Source: CAD feature listing. Evaluate the final solid. Frame: model axes, mm. A direction names the side the tool comes from. Coordinates: 2 decimals unless noted, no trailing zeros. Loops run counter-clockwise (first coordinate to the right, second up) from the corner with the lowest first, then second, coordinate; pieces in that order, holes last. Notation, with made-up numbers: M 24.25,-7.5 L 67.25,-7.5 A20 cw 67.25,8.5 Z; hole C 84.5,-22 d9. An arc over 180 degrees is marked long. One line per question, with ' | ' between items. Start each with the question number.
1. Section query B-B, the plane y = 13.15. Output: boundary loops of the cut face in (x, z) (3 decimals), and give its area (3 significant figures).
2. Pin query (flat end, axial travel): P1, Ø1.5, axis at x = -18, z = 18.5, coming from the +Y side; P2, Ø22.5, axis at x = 8.5, z = 4.5, coming from the +Y side; P3, Ø12, axis at x = -4.5, y = 71, coming from the +Z side. Return the tip coordinate at first contact, or that it passes through.
3. Section query C-C, the plane x = 25. Output: boundary loops of the cut face in (y, z) (3 decimals), and give its area (3 significant figures).
4. Section query A-A, the plane z = 7.5. Output: boundary loops of the cut face in (x, y).
5. Ray query, probe 1 along Z at (x, y) = (24.5, 22.4) (3 decimals); probe 2 along Y at (x, z) = (24.5, 0); probe 3 along Z at (x, y) = (33, 13). Return the intervals inside material, ascending.
6. Access query for faces 4 (the flat face through (20.3, 17, 10)), 5 (the flat face through (33, 25.4, 12)), 6 (the flat face through (15, 15, 10)), 7 (the flat face through (10, 127.3, 60)), 8 (the flat face through (-14, 16, 18)). Directions: +Z, -Z, +X, -X, +Y, -Y. A direction counts if a zero-diameter tool reaches every point of the face in a straight line with its end or side. Return the directions, or none.
7. Mould query, pull axis Z, two halves, no side actions, for faces 1 (the flat face through (10.3, 17, 10)), 2 (the flat face through (10, 65, 45)), 3 (the flat face through (-28, 8, 2)). Classes: pulls with the +Z half, pulls with the -Z half, needs draft (parallel to the pull), parting line crosses it, or undercut.
8. Section query D-D, the plane z = 25.5. Output: boundary loops of the cut face in (x, y), and give its area (3 significant figures).
```python
from build123d import *

# Parameters (mm, degrees)
SKETCH1_R           = 1.5
BOSS_EXTRUDE1_DEPTH = 5
BOSS_EXTRUDE2_START = 5
SKETCH1_4_R         = 1.5
BOSS_EXTRUDE2_DEPTH = 10.3
BOSS_EXTRUDE3_START = 15.3
SKETCH1_5_W         = 10.3
SKETCH1_5_H         = 5
SKETCH1_5_R         = 1.5
BOSS_EXTRUDE3_DEPTH = 5
SKETCH2_W           = 28
SKETCH2_H           = 16
SKETCH2_R           = 1.625
BOSS_EXTRUDE4_DEPTH = 5
BOSS_EXTRUDE5_START = 15.35
SKETCH2_2_W         = 28
SKETCH2_2_H         = 16
SKETCH2_2_R         = 1.625
BOSS_EXTRUDE5_DEPTH = 5
CUT_EXTRUDE1_START  = 127.3
SKETCH3_R           = 3.81
CUT_EXTRUDE1_DEPTH  = 12.7
BOSS_EXTRUDE6_START = 20.3
SKETCH1_6_R         = 1.5
BOSS_EXTRUDE6_DEPTH = 25
BOSS_EXTRUDE7_START = 10.3
SKETCH1_7_W         = 10.3
SKETCH1_7_H         = 3.4
BOSS_EXTRUDE7_DEPTH = 5
BOSS_EXTRUDE8_DEPTH = 20


with BuildPart() as part:
    # Sketch1 → Boss-Extrude1 (new body)
    with BuildSketch(Plane(origin=(0, 0, 0), x_dir=(0, 0, -1), z_dir=(1, 0, 0))):
        Polygon((-15.35, 0), (-15.35, 23.4), (-5.05, 23.4), (-5.05, 0), (5, 0), (5, 35.4), (-30, 35.4), (-30, 140), (-75, 140), (-75, 127.3), (-45, 127.3), (-45, 0), align=None)
        with Locations((-0.195, 2.4)):
            Circle(SKETCH1_R, mode=Mode.SUBTRACT)
        with Locations((-0.195, 22.4)):
            Circle(SKETCH1_R, mode=Mode.SUBTRACT)
        with Locations((-20.195, 22.4)):
            Circle(SKETCH1_R, mode=Mode.SUBTRACT)
        with Locations((-20.195, 2.4)):
            Circle(SKETCH1_R, mode=Mode.SUBTRACT)
    extrude(amount=BOSS_EXTRUDE1_DEPTH)

    # Sketch1<4> → Boss-Extrude2 (add)
    with BuildSketch(Plane(origin=(0, 0, 0), x_dir=(0, 0, -1), z_dir=(1, 0, 0)).offset(BOSS_EXTRUDE2_START)):
        Polygon((-5.05, 0), (5, 0), (5, 25.4), (-30, 25.4), (-30, 140), (-75, 140), (-75, 127.3), (-45, 127.3), (-45, 0), (-15.35, 0), (-15.35, 23.4), (-5.05, 23.4), align=None)
        with Locations((-0.195, 22.4)):
            Circle(SKETCH1_4_R, mode=Mode.SUBTRACT)
        with Locations((-0.195, 2.4)):
            Circle(SKETCH1_4_R, mode=Mode.SUBTRACT)
        with Locations((-20.195, 2.4)):
            Circle(SKETCH1_4_R, mode=Mode.SUBTRACT)
        with Locations((-20.195, 22.4)):
            Circle(SKETCH1_4_R, mode=Mode.SUBTRACT)
    extrude(amount=BOSS_EXTRUDE2_DEPTH)

    # Sketch1<5> → Boss-Extrude3 (add)
    with BuildSketch(Plane(origin=(0, 0, 0), x_dir=(0, 0, -1), z_dir=(1, 0, 0)).offset(BOSS_EXTRUDE3_START)):
        Polygon((-15.35, 0), (-15.35, 15), (-5.05, 15), (-5.05, 0), (5, 0), (5, 35.4), (-30, 35.4), (-30, 140), (-75, 140), (-75, 127.3), (-45, 127.3), (-45, 0), align=None)
        with Locations((-10.2, 20.9)):
            Rectangle(SKETCH1_5_W, SKETCH1_5_H, mode=Mode.SUBTRACT)
        with Locations(Location((-0.195, 2.4, 0), (0, 0, 180))):
            Circle(SKETCH1_5_R, mode=Mode.SUBTRACT)
        with Locations(Location((-0.195, 22.4, 0), (0, 0, 180))):
            Circle(SKETCH1_5_R, mode=Mode.SUBTRACT)
        with Locations(Location((-20.195, 22.4, 0), (0, 0, 180))):
            Circle(SKETCH1_5_R, mode=Mode.SUBTRACT)
        with Locations(Location((-20.195, 2.4, 0), (0, 0, 180))):
            Circle(SKETCH1_5_R, mode=Mode.SUBTRACT)
    extrude(amount=BOSS_EXTRUDE3_DEPTH)

    # Sketch2 → Boss-Extrude4 (add)
    with BuildSketch(Plane.XY):
        with Locations((-14, 8)):
            Rectangle(SKETCH2_W, SKETCH2_H)
        with Locations((-2.9, 2.85)):
            Circle(SKETCH2_R, mode=Mode.SUBTRACT)
        with Locations((-25.1, 13.15)):
            Circle(SKETCH2_R, mode=Mode.SUBTRACT)
    extrude(amount=BOSS_EXTRUDE4_DEPTH)

    # Sketch2<2> → Boss-Extrude5 (add)
    with BuildSketch(Plane.XY.offset(BOSS_EXTRUDE5_START)):
        with Locations((-14, 8)):
            Rectangle(SKETCH2_2_W, SKETCH2_2_H)
        with Locations((-2.9, 2.85)):
            Circle(SKETCH2_2_R, mode=Mode.SUBTRACT)
        with Locations((-25.1, 13.15)):
            Circle(SKETCH2_2_R, mode=Mode.SUBTRACT)
    extrude(amount=BOSS_EXTRUDE5_DEPTH)

    # Sketch3 → Cut-Extrude1 (cut)
    with BuildSketch(Plane(origin=(0, 0, 0), x_dir=(1, 0, 0), z_dir=(0, 1, 0)).offset(CUT_EXTRUDE1_START)):
        with Locations(Location((10.15, -55.95, 0), (0, 0, 90))):
            Circle(SKETCH3_R)
    extrude(amount=CUT_EXTRUDE1_DEPTH, mode=Mode.SUBTRACT)

    # Sketch1<6> → Boss-Extrude6 (add)
    with BuildSketch(Plane(origin=(0, 0, 0), x_dir=(0, 0, -1), z_dir=(1, 0, 0)).offset(BOSS_EXTRUDE6_START)):
        Polygon((-5.05, 0), (5, 0), (5, 25.4), (-30, 25.4), (-30, 0), (-15.35, 0), (-15.35, 23.4), (-5.05, 23.4), align=None)
        with Locations(Location((-0.195, 22.4, 0), (0, 0, 180))):
            Circle(SKETCH1_6_R, mode=Mode.SUBTRACT)
        with Locations(Location((-0.195, 2.4, 0), (0, 0, 180))):
            Circle(SKETCH1_6_R, mode=Mode.SUBTRACT)
        with Locations(Location((-20.195, 2.4, 0), (0, 0, 180))):
            Circle(SKETCH1_6_R, mode=Mode.SUBTRACT)
        with Locations(Location((-20.195, 22.4, 0), (0, 0, 180))):
            Circle(SKETCH1_6_R, mode=Mode.SUBTRACT)
    extrude(amount=BOSS_EXTRUDE6_DEPTH)

    # Sketch1<7> → Boss-Extrude7 (add)
    with BuildSketch(Plane(origin=(0, 0, 0), x_dir=(0, 0, -1), z_dir=(1, 0, 0)).offset(BOSS_EXTRUDE7_START)):
        with Locations((-10.2, 16.7)):
            Rectangle(SKETCH1_7_W, SKETCH1_7_H)
    extrude(amount=BOSS_EXTRUDE7_DEPTH)

    # Sketch1<9> → Boss-Extrude8 (add)
    with BuildSketch(Plane(origin=(0, 0, 0), x_dir=(0, 0, -1), z_dir=(1, 0, 0))):
        Polygon((-30, 25.4), (0, 25.4), (5, 25.4), (5, 35.4), (-30, 35.4), align=None)
    extrude(amount=BOSS_EXTRUDE8_DEPTH)


solid = part.part
```
Taken from the geometry:
1) outline: M -28,0 L -26.725,0 L -26.725,5 L -28,5 Z; M -28,15.35 L -26.725,15.35 L -26.725,20.35 L -28,20.35 Z; M -23.475,0 L 0,0 L 0,-5 L 45.3,-5 L 45.3,5.05 L 0,5.05 L 0,5 L -23.475,5 Z; M -23.475,15.35 L 45.3,15.35 L 45.3,30 L 20.3,30 L 20.3,45 L 0,45 L 0,20.35 L -23.475,20.35 Z | area: 1,670 mm^2
2) P1: y = 16 | P2: y = 35.4 | P3: z = 45
3) outline: M 0,-5 L 25.4,-5 L 25.4,30 L 0,30 L 0,15.35 L 23.4,15.35 L 23.4,5.05 L 0,5.05 Z; hole C 2.4,0.195 d3; hole C 2.4,20.195 d3; hole C 22.4,0.195 d3; hole C 22.4,20.195 d3 | area: 620 mm^2
4) outline: M 0,23.4 L 45.3,23.4 L 45.3,25.4 L 20.3,25.4 L 20.3,35.4 L 0,35.4 Z; M 10.3,15 L 20.3,15 L 20.3,18.4 L 10.3,18.4 Z
5) probe 1: -5 to -1.305, 1.695 to 5.05, 15.35 to 18.695, 21.695 to 30 | probe 2: 0 to 0.91, 3.89 to 20.91, 23.89 to 25.4 | probe 3: -5 to 5.05, 15.35 to 30
6) face 4: +X, -Y | face 5: +Z, -Z, +X, +Y | face 6: +X, -X, -Y | face 7: +Z, +X, -X, -Y | face 8: +Z, -Z, -X, +Y
7) face 1: undercut | face 2: pulls with the +Z half | face 3: needs draft
8) outline: M 0,0 L 45.3,0 L 45.3,25.4 L 20.3,25.4 L 20.3,35.4 L 0,35.4 Z | area: 1,350 mm^2
